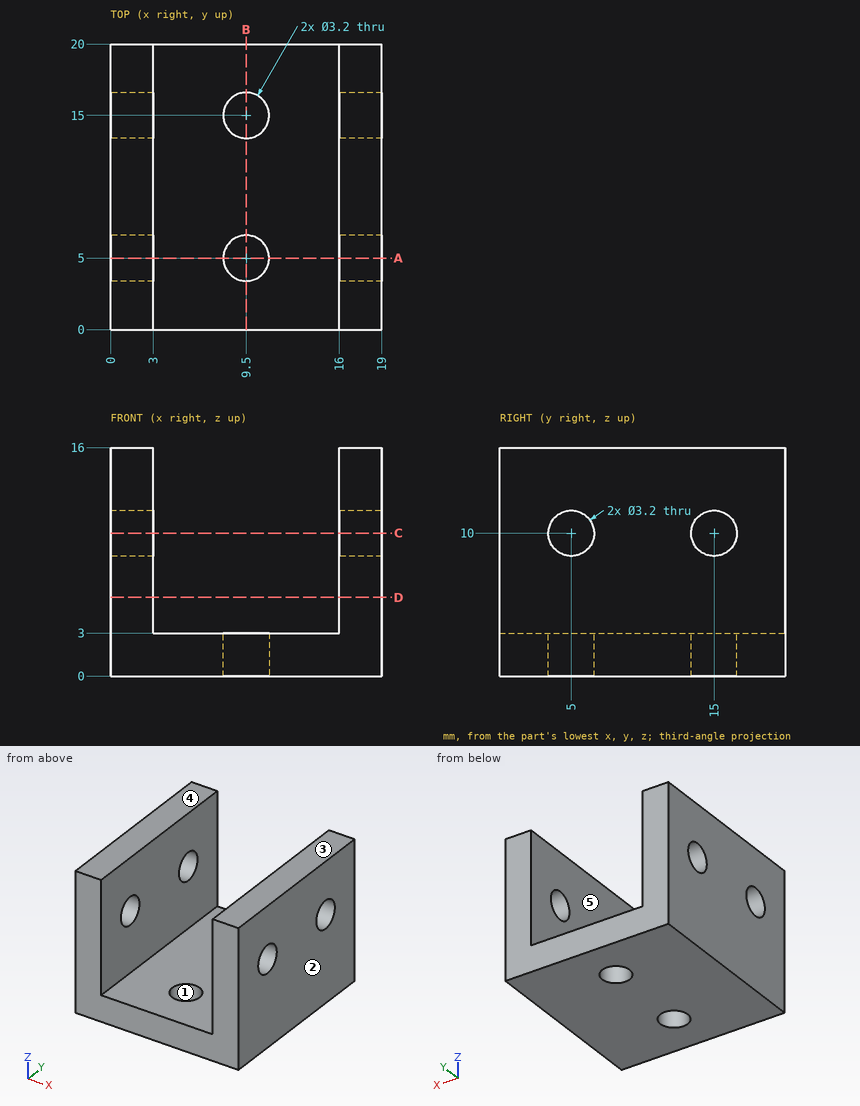
Answer from the drawing. Dimensions are ordinates in mm from the lowest x, y and z of the part. A direction names the side the tool comes from. Give positions to 0.01 mm unless a question says otherwise; leave off trailing zeros. Order: outer loops, then holes, each group sorted by start corner. A loop starts at its lowest first (then second) coordinate and runs counter-clockwise, first axis right, second up. Notation, with made-up numbers: (40.5, 63.25) - (89.5, 63.25) arc R17 ccw to (89.5, 73.25) - close; hole circle Ø11 at (-17, 16). An arc over 180 degrees is marked (long way). One line per item, written item: value. Start each with the question number.
1. Which of the six approach directions +Z, -Z, +X, -X, +Y, -Y give full straight-line access (tool end or side, diameter ignored) to the marked faces 4 and 5?
2. Section B-B, the plane x = 9.5 is taken. Write down the section's boundary in (y, z), then the cut area to 3 significant figures.
3. For a pull along X with two mould halves and no side action, classify the marked faces 1, 2 and 3 as released by +X, released by -X, zero draft, split by the parting line, or undercut.
4. Section D-D, the plane z = 5.5 is taken. Write down the section's boundary in (x, y), then the cut area to 3 significant figures.
5. Section C-C, the plane z = 10 is taken. Write down the section's boundary in (x, y).
6. Each of these flat-tipped pins is pushed along its axis until it touches: pin 1 Ø1.9 at (x, y) = (9.5, 5) entering from -Z; pin 2 Ø5 at (x, y) = (11, 9) entering from -Z; pin 3 Ø10.5 at (x, y) = (9, 8.5) entering from +Z. Where does it stop, or does it pass through?
7. Section A-A, the plane y = 5 is taken. Write down the section's boundary in (x, z), then the cut area to 3 significant figures.
8. Consider line 1 (Y direction, x = 18.35, z = 10); line 2 (X direction, y = 19.25, z = 5.75); line 3 (Z direction, x = 6, y = 2.25). Determine where each line is inside the solid, lowest interval first.
Filled sheet:
1. face 4: +Z, +X, -X, +Y, -Y
1. face 5: +Z, +Y, -Y
2. outline: (0, 0) - (3.4, 0) - (3.4, 3) - (0, 3) - close; (6.6, 0) - (13.4, 0) - (13.4, 3) - (6.6, 3) - close; (16.6, 0) - (20, 0) - (20, 3) - (16.6, 3) - close
2. area: 40.8 mm²
3. face 1: undercut
3. face 2: released by +X
3. face 3: zero draft
4. outline: (0, 0) - (3, 0) - (3, 20) - (0, 20) - close; (16, 0) - (19, 0) - (19, 20) - (16, 20) - close
4. area: 120 mm²
5. outline: (0, 0) - (3, 0) - (3, 3.4) - (0, 3.4) - close; (0, 6.6) - (3, 6.6) - (3, 13.4) - (0, 13.4) - close; (0, 16.6) - (3, 16.6) - (3, 20) - (0, 20) - close; (16, 0) - (19, 0) - (19, 3.4) - (16, 3.4) - close; (16, 6.6) - (19, 6.6) - (19, 13.4) - (16, 13.4) - close; (16, 16.6) - (19, 16.6) - (19, 20) - (16, 20) - close
6. pin 1: through
6. pin 2: z = 0
6. pin 3: z = 3
7. outline: (0, 0) - (7.9, 0) - (7.9, 3) - (3, 3) - (3, 8.4) - (0, 8.4) - close; (0, 11.6) - (3, 11.6) - (3, 16) - (0, 16) - close; (11.1, 0) - (19, 0) - (19, 8.4) - (16, 8.4) - (16, 3) - (11.1, 3) - close; (16, 11.6) - (19, 11.6) - (19, 16) - (16, 16) - close
7. area: 106 mm²
8. line 1: 0 to 3.4, 6.6 to 13.4, 16.6 to 20
8. line 2: 0 to 3, 16 to 19
8. line 3: 0 to 3
